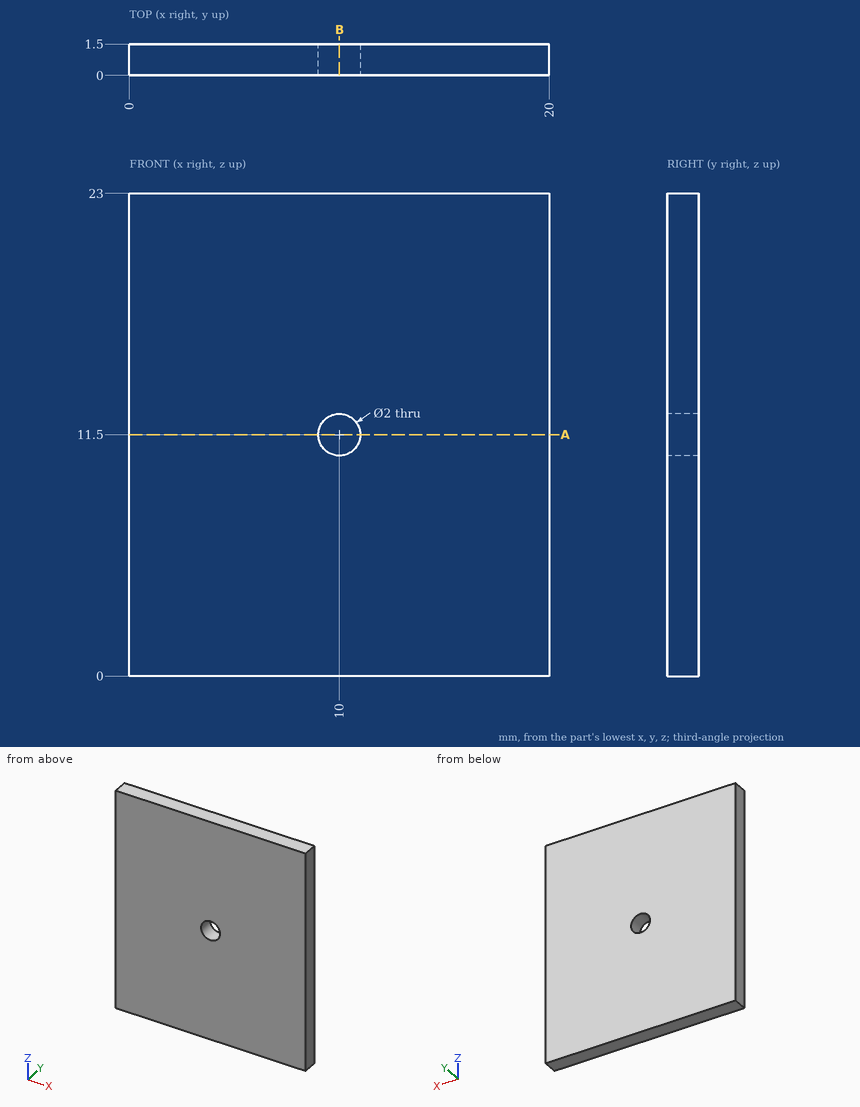
Can you work these out from the drawing? Everything is in mm from the part's minimum corner. Give positions to 0.01 mm unless a question says otherwise; leave off trailing zeros. Order: outer loops, then holes, each group sorted by start corner. A loop starts at its lowest first (then second) coordinate and runs counter-clockwise, first axis right, second up.
1. I need wall thicknesses on L1, parallel to Z at x = 10, y = 1.1. Which ranges of the line are inside material? Lowest first, please.
2. Suppose I cut it at A-A (z = 11.5). List the corners of the cut face in (x, y) for me, plus the area to 3 significant figures.
3. Suppose I cut it at B-B (x = 10). List the corners of the cut face in (y, z) for me, plus the area to 3 significant figures.
Solved:
1. L1: z = 0 to 10.5, 12.5 to 23
2. outline: (0, 0) - (9, 0) - (9, 1.5) - (0, 1.5) - close; (11, 0) - (20, 0) - (20, 1.5) - (11, 1.5) - close
2. area: 27.0 mm2
3. outline: (0, 0) - (1.5, 0) - (1.5, 10.5) - (0, 10.5) - close; (0, 12.5) - (1.5, 12.5) - (1.5, 23) - (0, 23) - close
3. area: 31.5 mm2
